Geometry: see drawing. Coordinates: mm, zero at the bounding-box minimum. A direction names the side the tool comes from. Coordinates: 2 decimals unless noted, no trailing zeros. Order: outer loops, then holes, each group sorted by start corner. A loop starts at its lowest first (then second) coordinate and runs counter-clockwise, first axis right, second up. Notation, with made-up numbers: M -28.75,80 L 17.25,80 A22 ccw 17.25,113 Z; hole C 13.25,1 d7. An arc over 180 degrees is marked long. Answer in a Markdown table with one row per item.
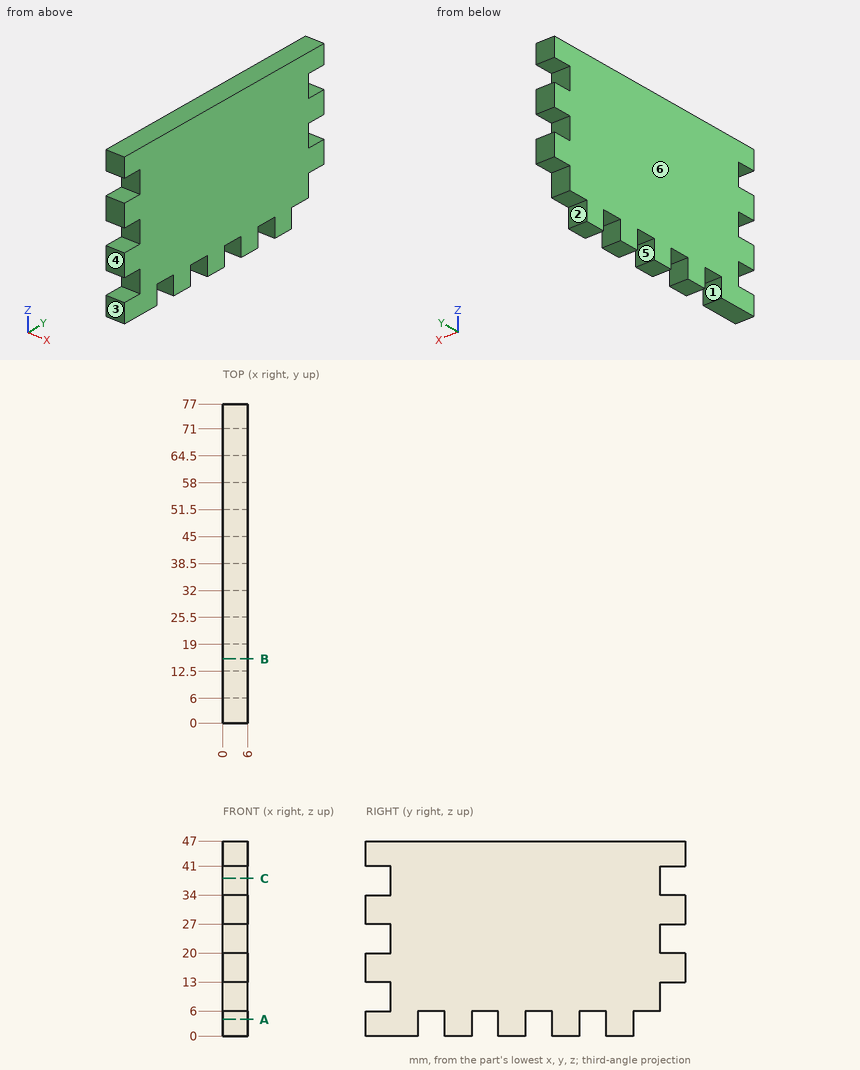
1) Material intervals for probe 1 along Y at (x, z) = (3.2, 24); probe 2 along Z at (x, y) = (0.85, 16), sorted ascending.
Resolved:
| item | result |
|---|---|
| probe 1 | y = 6 to 71 |
| probe 2 | z = 6 to 47 |
2) Cut plane C-C, the plane z = 38. Output: boundary loops of the cut face in (x, y), and give its area (3 significant figures).
Resolved:
| item | result |
|---|---|
| outline | M 0,6 L 6,6 L 6,71 L 0,71 Z |
| area | 390 mm2 |
3) Reachability of the marked faces 1, 2 and 3 from +Z, -Z, +X, -X, +Y, -Y: full face, straight path, thin tool, end or side. Return the list, or none.
Resolved:
| item | result |
|---|---|
| face 1 | -Z, +X, -X |
| face 2 | -Z, +X, -X, +Y |
| face 3 | +Z, -Z, +X, -X, -Y |
4) Cut plane B-B, the plane y = 15.5. Output: boundary loops of the cut face in (x, z), and give its area (3 significant figures).
Resolved:
| item | result |
|---|---|
| outline | M 0,6 L 6,6 L 6,47 L 0,47 Z |
| area | 246 mm2 |
5) Cut plane A-A, the plane z = 4. Output: boundary loops of the cut face in (x, y).
Resolved:
| item | result |
|---|---|
| outline | M 0,0 L 6,0 L 6,12.5 L 0,12.5 Z; M 0,19 L 6,19 L 6,25.5 L 0,25.5 Z; M 0,32 L 6,32 L 6,38.5 L 0,38.5 Z; M 0,45 L 6,45 L 6,51.5 L 0,51.5 Z; M 0,58 L 6,58 L 6,64.5 L 0,64.5 Z |
6) Contact query for flat-ended pins moving along their axis: pin 1 (1.8 mm diameter, centred on x = 2.5, y = 66, fed in from -Z); pin 2 (3 mm diameter, centred on x = 3.5, z = 4.5, fed in from -Y); pin 3 (3 mm diameter, centred on x = 2.5, z = 25, fed in from +Y); pin 4 (3 mm diameter, centred on x = 2.5, y = 74, fed in from -Z). Output: stop coordinate, or through.
Resolved:
| item | result |
|---|---|
| pin 1 | stops at z = 6 |
| pin 2 | stops at y = 0 |
| pin 3 | stops at y = 71 |
| pin 4 | stops at z = 13 |
7) Mould query, pull axis Y, two halves, no side actions, for the marked faces 4, 5 and 6. Classes: +Y half, -Y half, draft (parallel to the pull), parting line (faces both ways), or undercut.
Resolved:
| item | result |
|---|---|
| face 4 | -Y half |
| face 5 | undercut |
| face 6 | draft |
